Read the model definition and answer for the solid it produces. Units are mm, in the model's axes. A direction names the side the tool comes from. Coordinates: 2 decimals unless noted, no trailing zeros. Order: outer loops, then holes, each group sorted by start corner. A loop starts at its lowest first (then second) coordinate and runs counter-clockwise, first axis right, second up. Notation, with made-up numbers: M -18,8 L -8,8 A22 cw -8,24 Z; hole C 48,53.25 d1. An arc over 180 degrees is marked long. Put each result on its own line as item: value.
from build123d import *

# Parameters (mm, degrees)
CROQUIS1_W                   = 15
CROQUIS1_H                   = 5.9
CROQUIS1_W_2                 = 0.64
CROQUIS1_H_2                 = 0.8
SALIENTE_EXTRUIR1_DEPTH      = 1
CROQUIS2_W                   = 15
CROQUIS2_H                   = 5.9
CROQUIS2_W_2                 = 13.5
CROQUIS2_H_2                 = 4.4
SALIENTE_EXTRUIR2_DEPTH      = 6
CORTAR_EXTRUIR1_DEPTH        = 9
CORTAR_EXTRUIR2_DEPTH        = 2
SALIENTE_EXTRUIR3_DEPTH      = 6.5
SALIENTE_EXTRUIR3_DEPTH_BACK = 3.4
CROQUIS5_W                   = 0.64
CROQUIS5_H                   = 0.8


with BuildPart() as part:
    # Croquis1 → Saliente-Extruir1 (new body)
    with BuildSketch(Plane(origin=(0, 0, 0), x_dir=(1, 0, 0), z_dir=(0, 1, 0))):
        with Locations((5.02, 0.42)):
            Rectangle(CROQUIS1_W, CROQUIS1_H)
        Rectangle(CROQUIS1_W_2, CROQUIS1_H_2, mode=Mode.SUBTRACT)
        with Locations((10.04, 0)):
            Rectangle(CROQUIS1_W_2, CROQUIS1_H_2, mode=Mode.SUBTRACT)
        with Locations((7.54, 0)):
            Rectangle(CROQUIS1_W_2, CROQUIS1_H_2, mode=Mode.SUBTRACT)
        with Locations((2.5, 0)):
            Rectangle(CROQUIS1_W_2, CROQUIS1_H_2, mode=Mode.SUBTRACT)
        with Locations((5.02, 0)):
            Rectangle(CROQUIS1_W_2, CROQUIS1_H_2, mode=Mode.SUBTRACT)
    extrude(amount=SALIENTE_EXTRUIR1_DEPTH)

    # Croquis2 → Saliente-Extruir2 (add)
    with BuildSketch(Plane(origin=(0, 1, 0), x_dir=(1, 0, 0), z_dir=(0, 1, 0))):
        with Locations((5.02, 0.42)):
            Rectangle(CROQUIS2_W, CROQUIS2_H)
        with Locations((5.02, 0.42)):
            Rectangle(CROQUIS2_W_2, CROQUIS2_H_2, mode=Mode.SUBTRACT)
    extrude(amount=SALIENTE_EXTRUIR2_DEPTH)

    # Croquis3 → Cortar-Extruir1 (cut)
    with BuildSketch(Plane.ZY.offset(2.48)):
        with BuildLine():
            Line((1.78, 7), (1.78, 4.35))
            ThreePointArc((1.78, 4.35), (1.604264069, 3.925735931), (1.18, 3.75))
            Line((1.18, 3.75), (0.78, 3.75))
            Line((0.78, 3.75), (0.78, 7))
            Line((0.78, 7), (1.78, 7))
        make_face()
    extrude(amount=-CORTAR_EXTRUIR1_DEPTH, mode=Mode.SUBTRACT)

    # Croquis4 → Cortar-Extruir2 (cut)
    with BuildSketch(Plane.XY.offset(2.53)):
        with BuildLine():
            Line((-0.48, 7), (-0.48, 3.85))
            ThreePointArc((-0.48, 3.85), (-0.304264069, 3.425735931), (0.12, 3.25))
            Line((0.12, 3.25), (1.02, 3.25))
            Line((1.02, 3.25), (1.02, 7))
            Line((1.02, 7), (-0.48, 7))
        make_face()
        with BuildLine():
            Line((10.52, 7), (9.02, 7))
            Line((9.02, 7), (9.02, 3.25))
            Line((9.02, 3.25), (9.92, 3.25))
            ThreePointArc((9.92, 3.25), (10.344264069, 3.425735931), (10.52, 3.85))
            Line((10.52, 3.85), (10.52, 7))
        make_face()
    extrude(amount=-CORTAR_EXTRUIR2_DEPTH, mode=Mode.SUBTRACT)

    # Croquis5 → Saliente-Extruir3 (add, two sides: drawn at the far end of the back side and taken through both)
    with BuildSketch(Plane(origin=(0, 0, 0), x_dir=(1, 0, 0), z_dir=(0, 1, 0)).offset(-SALIENTE_EXTRUIR3_DEPTH_BACK)):
        with Locations((10.04, 0)):
            Rectangle(CROQUIS5_W, CROQUIS5_H)
        Rectangle(CROQUIS5_W, CROQUIS5_H)
        with Locations((2.5, 0)):
            Rectangle(CROQUIS5_W, CROQUIS5_H)
        with Locations((7.54, 0)):
            Rectangle(CROQUIS5_W, CROQUIS5_H)
        with Locations((5.02, 0)):
            Rectangle(CROQUIS5_W, CROQUIS5_H)
    extrude(amount=SALIENTE_EXTRUIR3_DEPTH + SALIENTE_EXTRUIR3_DEPTH_BACK)


solid = part.part
Q1. Given pin 1 (0.7 mm diameter, centred on x = 0, y = -1, fed in from -Z); pin 2 (0.7 mm diameter, centred on x = 7.5, z = 0, fed in from +Y); pin 3 (0.6 mm diameter, centred on y = -2, z = 0, fed in from -X), each flat-ended and moving along its own axis, determine where each tip first touches the part or whether it passes through.
Answers below:
pin 1: stops at z = -0.4
pin 2: stops at y = 6.5
pin 3: stops at x = -0.32
Q2. Consider line 1 along Z through (x, y) = (4, 3.5); line 2 along X through (y, z) = (3.5, -1.95); line 3 along Z through (x, y) = (0.25, 5.5). Determine where each line is inside the solid, lowest interval first.
Answers below:
line 1: z = -3.37 to -2.62, 1.78 to 2.53
line 2: x = -2.48 to -1.73, 11.77 to 12.52
line 3: z = -3.37 to -2.62, -0.4 to 0.4
Q3. Find section A-A on y = 2. Write down the section's boundary in (x, z).
Answers below:
outline: M -2.48,-3.37 L 12.52,-3.37 L 12.52,2.53 L -2.48,2.53 Z; M -0.32,-0.4 L 0.32,-0.4 L 0.32,0.4 L -0.32,0.4 Z; M 2.18,-0.4 L 2.82,-0.4 L 2.82,0.4 L 2.18,0.4 Z; M 4.7,-0.4 L 5.34,-0.4 L 5.34,0.4 L 4.7,0.4 Z; M 7.22,-0.4 L 7.86,-0.4 L 7.86,0.4 L 7.22,0.4 Z; M 9.72,-0.4 L 10.36,-0.4 L 10.36,0.4 L 9.72,0.4 Z; hole M -1.73,-2.62 L 11.77,-2.62 L 11.77,1.78 L -1.73,1.78 Z
Q4. Find section D-D on x = 9.25. Write down the section's boundary in (y, z), plus the area to 3 significant figures.
Answers below:
outline: M 0,-3.37 L 7,-3.37 L 7,-2.62 L 1,-2.62 L 1,1.78 L 3.25,1.78 L 3.25,2.53 L 0,2.53 Z
area: 12.1 mm^2
Q5. For a pull along X with two mould halves and no side action, classify faces 3 (the face through (-2.48, 3, 0)), 4 (the face through (5, 3, -3.37)), 5 (the face through (5, 4, -2.62)) as +X half, -X half, draft (parallel to the pull), parting line (faces both ways), or undercut.
Answers below:
face 3: -X half
face 4: draft
face 5: undercut
Q6. A tool of negligible diameter and unlimited length cuts with its end or side. For faces 1 (the face through (5, 4, 1.78)), 2 (the face through (12.52, 3, 0)), from which of +Z, -Z, +X, -X, +Y, -Y can it reach the whole face along a straight path? Write none if from no direction.
Answers below:
face 1: +Y
face 2: +Z, -Z, +X, +Y, -Y
Q7. Find section C-C on z = -1.4. Write down the section's boundary in (x, y), plus the area to 3 significant figures.
Answers below:
outline: M -2.48,0 L 12.52,0 L 12.52,7 L 11.77,7 L 11.77,1 L -1.73,1 L -1.73,7 L -2.48,7 Z
area: 24.0 mm^2
Q8. Find section B-B on y = -1. Write down the section's boundary in (x, z), plus the area to 3 significant figures.
Answers below:
outline: M -0.32,-0.4 L 0.32,-0.4 L 0.32,0.4 L -0.32,0.4 Z; M 2.18,-0.4 L 2.82,-0.4 L 2.82,0.4 L 2.18,0.4 Z; M 4.7,-0.4 L 5.34,-0.4 L 5.34,0.4 L 4.7,0.4 Z; M 7.22,-0.4 L 7.86,-0.4 L 7.86,0.4 L 7.22,0.4 Z; M 9.72,-0.4 L 10.36,-0.4 L 10.36,0.4 L 9.72,0.4 Z
area: 2.56 mm^2
